Here's how the part is built. I have some questions about the finished solid (model axes, mm). A direction names the side the tool comes from. Coordinates: 2 decimals unless noted, no trailing zeros. Write each loop counter-clockwise with the first axis right and the second up, starting at its lowest first coordinate (ties: lowest second). Pieces come first, ordered by that corner, then holes. Notation, with made-up numbers: (52.5, 23.25) -> (81.5, 23.25) arc R25 cw to (81.5, 50.25) -> close; hole circle Ø10 at (87, 8). An arc over 180 degrees is marked (long way). Put each result on its own line as item: value. Start each with the question number.
Item 1: If we mould it in two halves opening along Z, with no side actions, what happens to faces 6 (the face through (-1.39, -10.61, -0.08)), 7 (the face through (-7.4, -6, 0)), 8 (the face through (-6.4, 2.1, 2.775)), 9 (the face through (-9, 0, -5.775))? For each: released by +Z, released by -Z, zero draft, split by the parting line, or undercut.
Item 2: I want a section at C-C, the plane x = -3.75. List the corners of the cut face in (y, z) for me (3 decimals), then the cut area to 3 significant figures.
Item 3: I want a section at A-A, the plane x = -1. List the corners of the cut face in (y, z) for me (3 decimals).
Item 4: On a 3-axis mill with a long thin cutter (end or side, diameter ignored), from which of +Z, -Z, +X, -X, +Y, -Y can I reach the whole of each face in a straight line? I mean faces 1 (the face through (-8.748, 0.187, 4.296)), 2 (the face through (-5.69, 9.86, -0.08)), 3 (the face through (-8.748, -0.187, -4.296)), 4 (the face through (-0.4, 10, 0)), 5 (the face through (-9.07, -5.38, 0.08)). Say none if no direction works.
Item 5: I want a section at D-D, the plane y = 0. List the corners of the cut face in (x, z) for me (3 decimals), then the cut area to 3 significant figures.
Item 6: For pin 1 (3 mm diameter, centred on y = -8.03, z = 0, fed in from +X); pin 2 (5 mm diameter, centred on y = -2, z = 1.5, fed in from +X); pin 3 (1.3 mm diameter, centred on y = 6.5, z = 0, fed in from -X), each with a flat end and sliding along its axis, tell me the tip position at first contact or that it passes through.
Item 7: I need wall thicknesses on line 1 (Y direction, x = -5.75, z = 1); line 2 (Z direction, x = -10, y = -8) (3 decimals); line 3 (Y direction, x = -5, z = 0). Which ranges of each line are inside material? Lowest first, please. Write a range as [from, to].
Item 8: I want a section at B-B, the plane z = 4.75. List the corners of the cut face in (x, y) for me, then the cut area to 3 significant figures.
Solid Edge part; units mm, degrees
sketch "Sketch1" plane through (0, 0, 0) normal (0, 0, 1) x (1, 0, 0)
  line L0 (0, -6.5) -> (0, -10.7)
  arc A0 (0, -10.7) -> (-2.4041, -10.4264) centre (0, 0) cw
  line L1 (-10.7, -9) -> (-2.4041, -10.4264)
  line L2 (-10.7, 0) -> (-10.7, -9)
  line L3 (-10.7, 0) -> (-10.7, 9)
  line L4 (-10.7, 9) -> (-2.4041, 10.4264)
  line L5 (0, 10.7) -> (0, 6.5)
  arc A1 (-2.4041, 10.4264) -> (0, 10.7) centre (0, 0) cw
  arc A2 (0, -6.5) -> (0, 6.5) centre (0, 0) cw
extrude "Protrusion1" add sketch "Sketch1" along normal mid plane 11.55
sketch "Sketch2" plane through (-5.35, 0, 5.775) normal (0, 0, 1) x (0.9855377, -0.1694562, 0)
  arc A0 (6.7554, -7.7169) -> (3.7899, 9.53) centre (5.2726, 0.9066) cw
  line L0 (3.7899, 9.53) -> (4.1712, 7.3126)
  arc A1 (4.1712, 7.3126) -> (6.3741, -5.4994) centre (5.2726, 0.9066) ccw
  line L1 (6.3741, -5.4994) -> (6.7554, -7.7169)
extrude "ExtrudedCutout_1" cut sketch "Sketch2" against normal blind 3
mirror "Mirror1" about plane through (0, 0, 0) normal (0, 0, 1) of "ExtrudedCutout_1"
sketch "Sketch3" plane through (0, 0, 0) normal (0, 0, -1) x (-1, 0, 0)
  line L0 (0.4, 6.4877) -> (0, 6.4877)
  line L1 (0, 6.4877) -> (0, 10.7)
  line L2 (0, 10.7) -> (0.4, 10.7)
  line L3 (0.4, 10.7) -> (0.4, 6.4877)
extrude "ExtrudedCutout_2" cut sketch "Sketch3" along normal mid plane 12.1654
mirror "Mirror2" about plane through (0, 0, 0) normal (0, 1, 0) of "ExtrudedCutout_2"
sketch "Sketch4" plane through (-0.4, 8.5901, 0) normal (1, 0, 0) x (0, 0, 1)
  circle A0 centre (0, 0.5624) radius 1.55
  circle A1 centre (0, 16.6178) radius 1.55
extrude "ExtrudedCutout_3" cut sketch "Sketch4" along normal mid plane 184.4666
sketch "Sketch5" plane through (-10.7, 0, 0) normal (-1, 0, 0) x (0, 1, 0)
  circle A0 centre (-8.0277, 0) radius 2.65
  circle A1 centre (8.0277, 0) radius 2.65
extrude "ExtrudedCutout_4" cut sketch "Sketch5" against normal blind 3.3
properties material "PLA"
Calculated:
1. face 6: zero draft
1. face 7: undercut
1. face 8: released by +Z
1. face 9: released by -Z
2. outline: (-10.195, -5.775) -> (-7.906, -5.775) -> (-7.906, -2.775) -> (-5.309, -2.775) -> (-5.309, 2.775) -> (-7.906, 2.775) -> (-7.906, 5.775) -> (-10.195, 5.775) -> close; (5.309, -2.775) -> (7.906, -2.775) -> (7.906, -5.775) -> (10.195, -5.775) -> (10.195, 5.775) -> (7.906, 5.775) -> (7.906, 2.775) -> (5.309, 2.775) -> close; hole circle Ø3.1 at (-8.028, 0); hole circle Ø3.1 at (8.028, 0)
2. area: 66.6 mm2
3. outline: (-10.653, -5.775) -> (-8.693, -5.775) -> (-8.693, -2.775) -> (-6.423, -2.775) -> (-6.423, 2.775) -> (-8.693, 2.775) -> (-8.693, 5.775) -> (-10.653, 5.775) -> close; (6.423, -2.775) -> (8.693, -2.775) -> (8.693, -5.775) -> (10.653, -5.775) -> (10.653, 5.775) -> (8.693, 5.775) -> (8.693, 2.775) -> (6.423, 2.775) -> close; hole circle Ø3.1 at (-8.028, 0); hole circle Ø3.1 at (8.028, 0)
4. face 1: +Z, +X
4. face 2: +Z, -Z, -X, +Y
4. face 3: -Z, +X
4. face 4: +Z, -Z, +X, +Y, -Y
4. face 5: -X
5. outline: (-10.7, -5.775) -> (-8.75, -5.775) -> (-8.75, -2.775) -> (-6.5, -2.775) -> (-6.5, 2.775) -> (-8.75, 2.775) -> (-8.75, 5.775) -> (-10.7, 5.775) -> close
5. area: 35.0 mm2
6. pin 1: passes through
6. pin 2: stops at x = -4.69
6. pin 3: stops at x = -7.4
7. line 1: y = [-9.85, -9.21], [-6.84, -3.03], [3.03, 6.84], [9.21, 9.85]
7. line 2: z = [-5.775, -2.65], [2.65, 5.775]
7. line 3: y = [-9.98, -9.58], [-6.48, -4.15], [4.15, 6.48], [9.58, 9.98]
8. outline: (-10.7, -9) -> (-2.4, -10.43) arc R10.7 ccw to (-0.4, -10.69) -> (-0.4, -8.74) arc R8.75 cw to (-0.4, 8.74) -> (-0.4, 10.69) arc R10.7 ccw to (-2.4, 10.43) -> (-10.7, 9) -> close
8. area: 90.3 mm2
